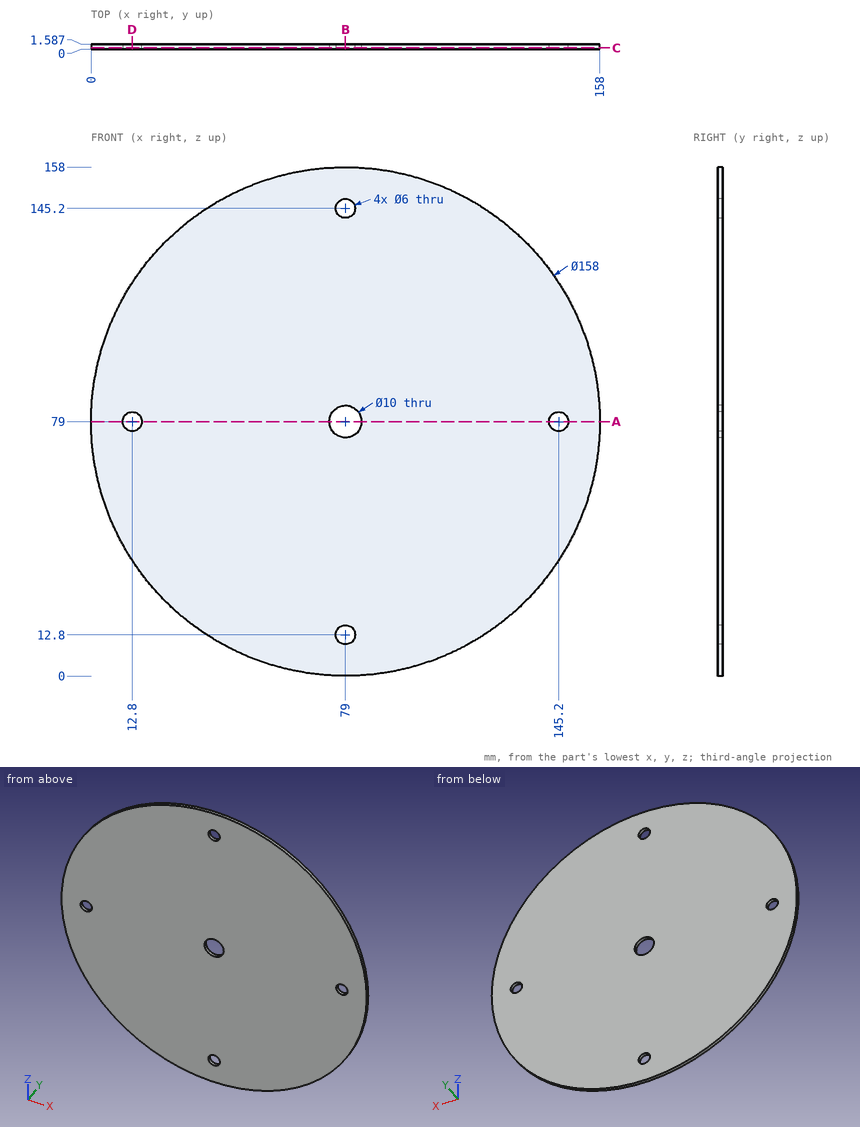
Source: three-view drawing plus pictorial views. Frame: mm from the lowest corner of the part. Coordinates: 2 decimals unless noted, no trailing zeros. Loops run counter-clockwise (first coordinate to the right, second up) from the corner with the lowest first, then second, coordinate; pieces in that order, holes last. Notation, with made-up numbers: (4, 4) - (58, 4) arc R22 ccw to (58, 28) - close; hole circle Ø8 at (51.25, 81.5). An arc over 180 degrees is marked (long way). Answer in a Markdown table with one row per item. Add a question column.
Item 1: Section query B-B on x = 79. Return the cut outline in (y, z).
Item 2: Line query: line 1 along Z through (x, y) = (79.5, 1.5) (1 decimal); line 2 along Z through (x, y) = (15, 0.4) (1 decimal). Output: solid intervals per line, ascending. Write a range as [from, to].
Item 3: Section query D-D on x = 12.8. Return the cut outline in (y, z).
Item 4: Section query A-A on z = 79. Return the cut outline in (x, y), then the cut area to 3 significant figures.
Item 5: Section query C-C on y = 0.4. Return the cut outline in (x, z).
Recorded:
| question | item | result |
|---|---|---|
| 1 | outline | (0, 0) - (1.59, 0) - (1.59, 9.8) - (0, 9.8) - close; (0, 15.8) - (1.59, 15.8) - (1.59, 74) - (0, 74) - close; (0, 84) - (1.59, 84) - (1.59, 142.2) - (0, 142.2) - close; (0, 148.2) - (1.59, 148.2) - (1.59, 158) - (0, 158) - close |
| 2 | line 1 | [0, 9.8], [15.8, 74], [84, 142.2], [148.2, 158] |
| 2 | line 2 | [32.7, 77], [81, 125.3] |
| 3 | outline | (0, 35.89) - (1.59, 35.89) - (1.59, 76) - (0, 76) - close; (0, 82) - (1.59, 82) - (1.59, 122.11) - (0, 122.11) - close |
| 4 | outline | (0, 0) - (9.8, 0) - (9.8, 1.59) - (0, 1.59) - close; (15.8, 0) - (74, 0) - (74, 1.59) - (15.8, 1.59) - close; (84, 0) - (142.2, 0) - (142.2, 1.59) - (84, 1.59) - close; (148.2, 0) - (158, 0) - (158, 1.59) - (148.2, 1.59) - close |
| 4 | area | 216 mm^2 |
| 5 | outline | circle Ø158 at (79, 79); hole circle Ø6 at (12.8, 79); hole circle Ø10 at (79, 79); hole circle Ø6 at (79, 12.8); hole circle Ø6 at (79, 145.2); hole circle Ø6 at (145.2, 79) |
